```python
from build123d import *

# Parameters (mm, degrees)
SKETCH1_R          = 7.9375
BASE_EXTRUDE_DEPTH = 4.6101


with BuildPart() as part:
    # Sketch1 → Base-Extrude (new, symmetric)
    with BuildSketch(Plane.XY):
        Polygon((13.748153285, 0), (6.874076643, 11.90625), (-6.874076643, 11.90625), (-13.748153285, 0), (-6.874076643, -11.90625), (6.874076643, -11.90625), align=None)
        Circle(SKETCH1_R, mode=Mode.SUBTRACT)
    extrude(amount=BASE_EXTRUDE_DEPTH, both=True)

    # Sketch2 → Cut-Revolve1 (revolve, cut)
    with BuildSketch(Plane(origin=(0, 0, 0), x_dir=(1, 0, 0), z_dir=(0, 1, 0))):
        with BuildLine():
            Line((13.748153285, 4.6101), (13.748153285, 1.84404))
            ThreePointArc((13.748153285, 1.84404), (12.937993068, 3.799939783), (10.982093285, 4.6101))
            Line((10.982093285, 4.6101), (13.748153285, 4.6101))
        make_face()
        with BuildLine():
            Line((13.748153285, -4.6101), (10.982093285, -4.6101))
            ThreePointArc((10.982093285, -4.6101), (12.937993068, -3.799939783), (13.748153285, -1.84404))
            Line((13.748153285, -1.84404), (13.748153285, -4.6101))
        make_face()
    revolve(axis=Axis((0, 0, 0), (0, 0, -1)), mode=Mode.SUBTRACT)


solid = part.part
```
Part model, mm, in its own coordinate system. Round coordinates to 2 decimals unless told otherwise and drop trailing zeros. Order: outer loops, then holes, each group sorted by start corner. A loop starts at its lowest first (then second) coordinate and runs counter-clockwise, first axis right, second up. Notation, with made-up numbers: M 29.25,-11 L 67.25,-11 A25 ccw 67.25,6 Z; hole C 81,24 d9. An arc over 180 degrees is marked long. Put each result on its own line as item: value. Start each with the question number.
1. Slice it at D-D on z = 4. List the corners of the cut face in (x, y) (1 decimal), then the cut area to 3 significant figures.
2. Slice it at B-B on z = -1.5. List the corners of the cut face in (x, y) (1 decimal).
3. Two-plate mould, pull along X, no slides. Class faces 1 (the face through (0, 11.906, 0)), 2 (the face through (-1.72, -7.75, -0.06)), 3 (the face through (-10.26, 6.04, 0.06)), 4 (the face through (10.26, -6.04, 0.06)): +X half, -X half, draft (parallel to the pull), parting line (faces both ways), or undercut.
4. Drop flat-ended pins along their axis: pin 1 (5 mm diameter, centred on y = -6.5, z = -2, fed in from +X); pin 2 (4 mm diameter, centred on x = 8, z = 3.5, fed in from -Y); pin 3 (3 mm diameter, centred on y = -7.5, z = 1, fed in from -X). Give the stop position or say it passes through.
5. Slice it at A-A on x = 0. List the corners of the cut face in (y, z).
6. Slice it at C-C on z = -3.25. List the corners of the cut face in (x, y) (1 decimal), then the cut area to 3 significant figures.
7. Drill centre lines: probe 1 along Y at (x, z) = (0, 0); probe 2 along X at (y, z) = (-2.5, -3.5); probe 3 along X at (y, z) = (-0.25, -1.75). Where is each one in solid material? Low to high. Write a range as [from, to].
Findings:
1. outline: M -12.5,-2.1 L -8.1,-9.8 A12.7 ccw -4.5,-11.9 L 4.5,-11.9 A12.7 ccw 8.1,-9.8 L 12.5,-2.1 A12.7 ccw 12.5,2.1 L 8.1,9.8 A12.7 ccw 4.5,11.9 L -4.5,11.9 A12.7 ccw -8.1,9.8 L -12.5,2.1 A12.7 ccw Z; hole C 0,0 d15.9
1. area: 281 mm2
2. outline: M -13.7,0 L -6.9,-11.9 L 6.9,-11.9 L 13.7,0 L 6.9,11.9 L -6.9,11.9 Z; hole C 0,0 d15.9
3. face 1: draft
3. face 2: undercut
3. face 3: -X half
3. face 4: +X half
4. pin 1: x = 11.44
4. pin 2: y = -11.91
4. pin 3: x = -10.28
5. outline: M -11.91,-4.45 A2.77 ccw -10.98,-4.61 L -7.94,-4.61 L -7.94,4.61 L -10.98,4.61 A2.77 ccw -11.91,4.45 Z; M 7.94,-4.61 L 10.98,-4.61 A2.77 ccw 11.91,-4.45 L 11.91,4.45 A2.77 ccw 10.98,4.61 L 7.94,4.61 Z
6. outline: M -13.3,-0.7 L -7.3,-11.2 A13.4 ccw -6.1,-11.9 L 6.1,-11.9 A13.4 ccw 7.3,-11.2 L 13.3,-0.7 A13.4 ccw 13.3,0.7 L 7.3,11.2 A13.4 ccw 6.1,11.9 L -6.1,11.9 A13.4 ccw -7.3,11.2 L -13.3,0.7 A13.4 ccw Z; hole C 0,0 d15.9
6. area: 292 mm2
7. probe 1: [-11.91, -7.94], [7.94, 11.91]
7. probe 2: [-12.3, -7.53], [7.53, 12.3]
7. probe 3: [-13.6, -7.93], [7.93, 13.6]
